Can you work these out from the model? Positions are in its coordinate system, mm. Give positions to 0.01 mm unless a question says otherwise; leave off trailing zeros. Loops run counter-clockwise (first coordinate to the right, second up) from the corner with the lowest first, then second, coordinate; pieces in that order, holes last. Notation, with made-up numbers: (18.5, 58.25) -> (68.5, 58.25) arc R8 cw to (68.5, 73.25) -> close; hole circle Ø7 at (40.5, 45.5). An arc over 180 degrees is marked (long way). Use CSV: the item, a comma, the result in double quotes.
from build123d import *

# Parameters (mm, degrees)
BOSS_EXTRUDE1_DEPTH = 2
BOSS_EXTRUDE2_DEPTH = 2.15


with BuildPart() as part:
    # Sketch1 → Boss-Extrude1 (new body)
    with BuildSketch(Plane(origin=(0, 0, 0), x_dir=(1, 0, 0), z_dir=(0, 1, 0))):
        with BuildLine():
            Line((-12.039826938, -3.360441535), (-6, -25))
            Line((-6, -25), (6, -25))
            Line((6, -25), (12.039826938, -3.360441535))
            ThreePointArc((12.039826938, -3.360441535), (0, 12.5), (-12.039826938, -3.360441535))
        make_face()
    extrude(amount=BOSS_EXTRUDE1_DEPTH)

    # Sketch2 → Boss-Extrude2 (add)
    with BuildSketch(Plane(origin=(0, 2, 0), x_dir=(1, 0, 0), z_dir=(0, 1, 0))):
        with BuildLine():
            Line((-6, -25), (-6, -12.093386622))
            ThreePointArc((-6, -12.093386622), (0, -13.5), (6, -12.093386622))
            Line((6, -12.093386622), (6, -25))
            Line((6, -25), (-6, -25))
        make_face()
    extrude(amount=BOSS_EXTRUDE2_DEPTH)


solid = part.part
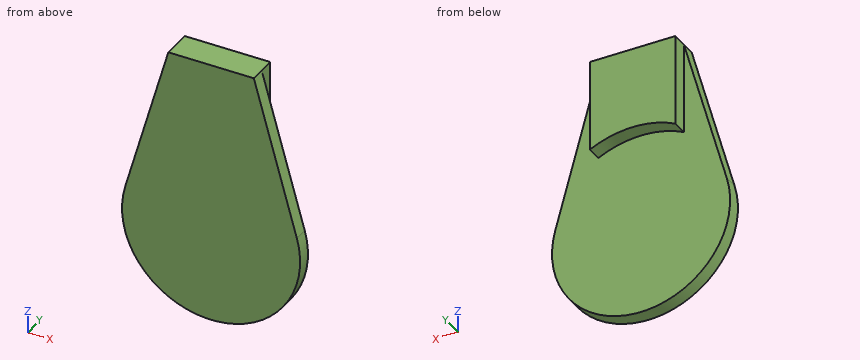
(1) If I drill on L1, parallel to Y at x = -10, z = 7.5; L2, parallel to X at y = 2.9, z = 20; L3, parallel to X at y = 1.7, z = -3, over which ranges is the centre line in solid material (lowest first)? Write a range as from..to.
Answer sheet:
L1,"y = 0..2"
L2,"x = -6..6"
L3,"x = -12.13..12.13"
(2) If we section it at D-D, the plane x = 4.5: Write out the boundary of the cut face in (y, z), then the cut area to 3 significant figures.
Answer sheet:
outline,"(0, -11.66) -> (2, -11.66) -> (2, 12.73) -> (4.15, 12.73) -> (4.15, 25) -> (0, 25) -> close"
area,"99.7 mm2"
(3) If we section it at A-A, the plane x = 0: Write out the boundary of the cut face in (y, z), then the cut area to 3 significant figures.
Answer sheet:
outline,"(0, -12.5) -> (2, -12.5) -> (2, 13.5) -> (4.15, 13.5) -> (4.15, 25) -> (0, 25) -> close"
area,"99.7 mm2"
(4) Will these pins go through, and if not, where does the flat tip stop? pin 1 Ø2 at (x, z) = (4.5, 4) entering from +Y; pin 2 Ø4 at (x, z) = (9, 9.5) entering from -Y; pin 3 Ø1.1 at (y, z) = (3.5, 18) entering from +X; pin 4 Ø1.1 at (y, z) = (3, 16) entering from -X.
Answer sheet:
pin 1,"stops at y = 2"
pin 2,"stops at y = 0"
pin 3,"stops at x = 6"
pin 4,"stops at x = -6"
(5) If we section it at B-B, the plane z = -10: Write out the boundary of the cut face in (x, y), then the cut area to 3 significant figures.
Answer sheet:
outline,"(-7.5, 0) -> (7.5, 0) -> (7.5, 2) -> (-7.5, 2) -> close"
area,"30.0 mm2"
(6) If we section it at C-C, the plane y = 2.6: Write out the boundary of the cut face in (x, z).
Answer sheet:
outline,"(-6, 12.09) arc R13.5 cw to (6, 12.09) -> (6, 25) -> (-6, 25) -> close"
